Input: part model. Units: mm. Frame: model coordinates. A direction names the side the tool comes from. Give positions to 0.01 mm unless a question says otherwise; leave off trailing zeros. Loops run counter-clockwise (first coordinate to the right, second up) from the corner with the lowest first, then second, coordinate; pieces in that order, holes last. Notation, with made-up numbers: (-34.5, 83) -> (-9.5, 83) arc R23 ccw to (-9.5, 101) -> close; hole circle Ø3 at (38, -23.5). An arc over 180 degrees is marked (long way). One line per question, with ' | ' between items.
from build123d import *

# Parameters (mm, degrees)
SKETCH1_W           = 1130
SKETCH1_H           = 500
BOSS_EXTRUDE1_DEPTH = 60
SKETCH2_W           = 1030
SKETCH2_H           = 400
CUT_EXTRUDE1_DEPTH  = 60
SKETCH3_W           = 50
SKETCH3_H           = 500
BOSS_EXTRUDE3_DEPTH = 700
SKETCH5_W           = 434.818131318
SKETCH5_H           = 650
CUT_EXTRUDE2_DEPTH  = 1902


with BuildPart() as part:
    # Sketch1 → Boss-Extrude1 (new body)
    with BuildSketch(Plane(origin=(0, 0, 0), x_dir=(1, 0, 0), z_dir=(0, 1, 0))):
        Rectangle(SKETCH1_W, SKETCH1_H)
    extrude(amount=BOSS_EXTRUDE1_DEPTH)

    # Sketch2 → Cut-Extrude1 (cut)
    with BuildSketch(Plane(origin=(0, 60, 0), x_dir=(1, 0, 0), z_dir=(0, 1, 0))):
        Rectangle(SKETCH2_W, SKETCH2_H)
    extrude(amount=-CUT_EXTRUDE1_DEPTH, mode=Mode.SUBTRACT)

    # Sketch3 → Boss-Extrude3 (add)
    with BuildSketch(Plane(origin=(0, 0, 0), x_dir=(-1, 0, 0), z_dir=(0, -1, 0))):
        with Locations((540, 0)):
            Rectangle(SKETCH3_W, SKETCH3_H)
        with Locations((-540, 0)):
            Rectangle(SKETCH3_W, SKETCH3_H)
    extrude(amount=BOSS_EXTRUDE3_DEPTH)

    # Sketch5 → Cut-Extrude2 (cut)
    with BuildSketch(Plane.ZY.offset(565)):
        with Locations((3.135707678, -325)):
            Rectangle(SKETCH5_W, SKETCH5_H)
    extrude(amount=-CUT_EXTRUDE2_DEPTH, mode=Mode.SUBTRACT)


solid = part.part
1. Section query C-C (x = -148). Output: boundary loops of the cut face in (y, z).
Determined:
outline: (0, -250) -> (60, -250) -> (60, -200) -> (0, -200) -> close; (0, 200) -> (60, 200) -> (60, 250) -> (0, 250) -> close
2. Section query A-A (y = -560). Output: boundary loops of the cut face in (x, z).
Determined:
outline: (-565, -250) -> (-515, -250) -> (-515, -214.27) -> (-565, -214.27) -> close; (-565, 220.54) -> (-515, 220.54) -> (-515, 250) -> (-565, 250) -> close; (515, -250) -> (565, -250) -> (565, -214.27) -> (515, -214.27) -> close; (515, 220.54) -> (565, 220.54) -> (565, 250) -> (515, 250) -> close
3. Ray query, line 1 along X through (y, z) = (19, -156.5); line 2 along Y through (x, z) = (-454, 210). Return the intervals inside material, ascending. Write a range as from..to.
Determined:
line 1: x = -565..-515, 515..565 | line 2: y = 0..60
4. Pull-direction query (Z, two-part tool) for faces 1 (the flat face through (44, 20, -250)), 2 (the flat face through (-540, -330, -214.273)), 3 (the flat face through (-515, -659, 1)), 4 (the flat face through (-540, -650, 0)); classes: pulls with the +Z half, pulls with the -Z half, needs draft (parallel to the pull), parting line crosses it, or undercut.
Determined:
face 1: pulls with the -Z half | face 2: undercut | face 3: needs draft | face 4: undercut
5. Section query B-B (z = -40). Output: boundary loops of the cut face in (x, y).
Determined:
outline: (-565, -700) -> (-515, -700) -> (-515, -650) -> (-565, -650) -> close; (-565, 0) -> (-515, 0) -> (-515, 60) -> (-565, 60) -> close; (515, -700) -> (565, -700) -> (565, -650) -> (515, -650) -> close; (515, 0) -> (565, 0) -> (565, 60) -> (515, 60) -> close
6. Reachability of faces 5 (the flat face through (-3, 0, -205)), 6 (the flat face through (-7, 30, -200)), 7 (the flat face through (-540, -330, 220.545)) from +Z, -Z, +X, -X, +Y, -Y: full face, straight path, thin tool, end or side. Return the list, or none.
Determined:
face 5: none | face 6: +Y, -Y | face 7: +X, -X
